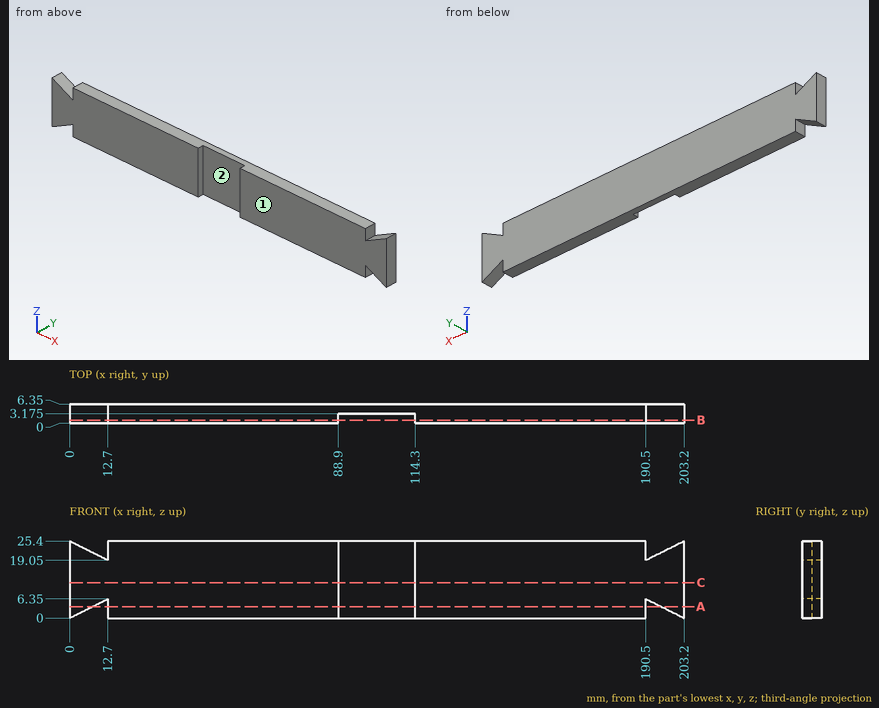
Check sheet for the drawn part. Datum: minimum x, y, z corner. Units: mm. A direction names the side the tool comes from. Coordinates: 2 decimals unless noted, no trailing zeros. Order: outer loops, then holes, each group sorted by start corner. A loop starts at its lowest first (then second) coordinate and runs counter-clockwise, first axis right, second up. Notation, with made-up numbers: M 46.5,57 L 103.5,57 A36 cw 103.5,92 Z; hole C 64.5,-36.75 d3. An arc over 180 degrees is marked long. One line per item, written item: value. Start each with the question number.
Item 1: Scan lines: probe 1 along X at (y, z) = (1.25, 7); probe 2 along X at (y, z) = (3.75, 3); probe 3 along X at (y, z) = (4.5, 4). Record each from-to range of solid material in increasing order.
Item 2: Sectioned sample at A-A (z = 3.75). Enter the section's corners in (x, y) (3 decimals).
Item 3: Access from +Z, -Z, +X, -X, +Y, -Y to the whole of each face (thin tool, end or side, straight path). Record for the marked faces 1 and 2.
Item 4: Sectioned sample at C-C (z = 11.75). Enter the section's corners in (x, y) (3 decimals), then the cut area to 3 significant figures.
Item 5: Gauge pin test, flat end, axial feed: pin 1 (6 mm diameter, centred on x = 100, z = 7.5, fed in from -Y) (3 decimals). Record the tip position at first contact, or that the pin passes through.
Item 6: Sectioned sample at B-B (y = 1). Enter the section's corners in (x, z), then the cut area to 3 significant figures.
Conclusion:
1. probe 1: x = 0 to 88.9, 114.3 to 203.2
1. probe 2: x = 0 to 6, 12.7 to 190.5, 197.2 to 203.2
1. probe 3: x = 0 to 8, 12.7 to 190.5, 195.2 to 203.2
2. outline: M 0,0 L 7.5,0 L 7.5,6.35 L 0,6.35 Z; M 12.7,0 L 88.9,0 L 88.9,3.175 L 114.3,3.175 L 114.3,0 L 190.5,0 L 190.5,6.35 L 12.7,6.35 Z; M 195.7,0 L 203.2,0 L 203.2,6.35 L 195.7,6.35 Z
3. face 1: +Z, -Z, +X, -X, -Y
3. face 2: +Z, -Z, -Y
4. outline: M 0,0 L 88.9,0 L 88.9,3.175 L 114.3,3.175 L 114.3,0 L 203.2,0 L 203.2,6.35 L 0,6.35 Z
4. area: 1,210 mm^2
5. pin 1: stops at y = 3.175
6. outline: M 0,0 L 12.7,6.35 L 12.7,0 L 88.9,0 L 88.9,25.4 L 12.7,25.4 L 12.7,19.05 L 0,25.4 Z; M 114.3,0 L 190.5,0 L 190.5,6.35 L 203.2,0 L 203.2,25.4 L 190.5,19.05 L 190.5,25.4 L 114.3,25.4 Z
6. area: 4,350 mm^2
